Part model, mm, in its own coordinate system. Give positions to 0.01 mm unless a question says otherwise; leave off trailing zeros. Write each loop counter-clockwise with the first axis right and the second up, starting at its lowest first coordinate (ties: lowest second). Pieces come first, ordered by that corner, then holes. Notation, with made-up numbers: (16.25, -28) - (37.25, -28) arc R19 ccw to (37.25, 6) - close; hole circle Ø8 at (60.25, 28). An arc over 180 degrees is marked (long way). Answer in a Markdown table with one row per item. Add a question column.
1. Pull direction X, two halves, no side cores. Call faces 1 (the flat face through (0, 32, 14)), 2 (the cylindrical face through (14.273, 55.007, 11.918)), 3 (the flat face through (4, 33, 0)), 4 (the cylindrical face through (13.727, 9.993, 8.918)): released by +X, released by -X, zero draft, split by the parting line, or undercut.
2. Drop a flat-ended pin along its axis: pin 1 Ø5 at (x, z) = (14, 14) entering from +Y. Give the stop position or say it passes through.
3. Band-saw the part on A-A on z = 17.75. Write the cut outline in (x, y), plus the area to 3 significant figures.
4. Band-saw the part on B-B on y = 57. Write the cut outline in (x, z).
5. Probe line 1 along X through (y, z) = (59.25, 14); line 2 along Y through (x, z) = (14, 7.5). List the from-to ranges inside material, lowest first.
```python
from build123d import *

# Parameters (mm, degrees)
SKETCH1_W             = 28
SKETCH1_H             = 65
SKETCH1_R             = 7.5
BOSS_EXTRUDE1_DEPTH   = 28
M5_TAPPED_HOLE3_D     = 4.2
M5_TAPPED_HOLE3_DEPTH = 18.7381927
M5_TAPPED_HOLE3_TIP   = 1.2618073
M5_TAPPED_HOLE4_D     = 4.2
M5_TAPPED_HOLE4_DEPTH = 18.7381927
M5_TAPPED_HOLE4_TIP   = 1.2618073
CHAMFER1_SIZE         = 1


with BuildPart() as part:
    # Sketch1 → Boss-Extrude1 (new body)
    with BuildSketch(Plane.XY):
        with Locations((14, 32.5)):
            Rectangle(SKETCH1_W, SKETCH1_H)
        with Locations((14, 32.5)):
            Circle(SKETCH1_R, mode=Mode.SUBTRACT)
    extrude(amount=BOSS_EXTRUDE1_DEPTH)

    # M5 Tapped Hole3
    with Locations(Plane(origin=(0, 0, 0), x_dir=(-1, 0, 0), z_dir=(0, -1, 0))):
        with Locations((-14, -11)):
            Hole(M5_TAPPED_HOLE3_D / 2, depth=M5_TAPPED_HOLE3_DEPTH)
            with Locations((0, 0, -(M5_TAPPED_HOLE3_DEPTH + M5_TAPPED_HOLE3_TIP / 2))):  # 118° drill point
                Cone(0, M5_TAPPED_HOLE3_D / 2, M5_TAPPED_HOLE3_TIP, mode=Mode.SUBTRACT)

    # M5 Tapped Hole4
    with Locations(Plane(origin=(0, 65, 0), x_dir=(1, 0, 0), z_dir=(0, 1, 0))):
        with Locations((14, -14)):
            Hole(M5_TAPPED_HOLE4_D / 2, depth=M5_TAPPED_HOLE4_DEPTH)
            with Locations((0, 0, -(M5_TAPPED_HOLE4_DEPTH + M5_TAPPED_HOLE4_TIP / 2))):  # 118° drill point
                Cone(0, M5_TAPPED_HOLE4_D / 2, M5_TAPPED_HOLE4_TIP, mode=Mode.SUBTRACT)

    # Chamfer1
    chamfer1_edges = [part.edges().sort_by_distance(p)[0] for p in [
        (6.5, 32.5, 0),
        (6.5, 32.5, 28),
        (11.9, 0, 11),
        (16.1, 65, 14),
    ]]
    chamfer(chamfer1_edges, length=CHAMFER1_SIZE)


solid = part.part
```
Values:
| question | item | result |
|---|---|---|
| 1 | face 1 | released by -X |
| 1 | face 2 | undercut |
| 1 | face 3 | zero draft |
| 1 | face 4 | undercut |
| 2 | pin 1 | stops at y = 64.4 |
| 3 | outline | (0, 0) - (28, 0) - (28, 65) - (0, 65) - close; hole circle Ø15 at (14, 32.5) |
| 3 | area | 1,640 mm² |
| 4 | outline | (0, 0) - (28, 0) - (28, 28) - (0, 28) - close; hole circle Ø4.2 at (14, 14) |
| 5 | line 1 | x = 0 to 11.9, 16.1 to 28 |
| 5 | line 2 | y = 0 to 25, 40 to 65 |
